Geometry check sheet. Reference: the model listing, model coordinates, mm. Face numbers are marked on the shaded views. Round coordinates to 2 decimals unless told otherwise and drop trailing zeros. Loops run counter-clockwise (first coordinate to the right, second up) from the corner with the lowest first, then second, coordinate; pieces in that order, holes last. Notation, with made-up numbers: (-20, -17.5) -> (12, -17.5) arc R23 cw to (12, 14.5) -> close; hole circle Ø10 at (75, -18). An arc over 180 degrees is marked (long way). Use a Markdown table: item, result. Add a question column.
Q1. Gauge pin test, flat ends, axial feed: P1, Ø6, axis at x = 12, z = 14.5, coming from the -Y side; P2, Ø13, axis at x = 5, y = 28, coming from the +Z side; P3, Ø8, axis at x = 25, y = 32.5, coming from the +Z side. Record the tip position at first contact, or that the pin passes through.
Q2. Sectioned sample at B-B, the plane z = 2. Enter the section's corners in (x, y).
Q3. Release check for a two-part mould opening along Y. For the marked faces 1, 2, 3 and 4 record: released by +Y, released by -Y, zero draft, split by the parting line, or undercut.
Q4. Sectioned sample at A-A, the plane x = 15. Enter the section's corners in (y, z), then the cut area to 3 significant figures.
Q5. Material ranges on L1, parallel to Z at x = 15, y = 33.5; L2, parallel to Y at x = 5, z = 1.5; L3, parallel to Y at x = 14, z = 15, recorded low to high.
Q6. Sectioned sample at D-D, the plane z = 19. Enter the section's corners in (x, y), then the cut area to 3 significant figures.
Q7. Sectioned sample at C-C, the plane y = 32. Enter the section's corners in (x, z), then the cut area to 3 significant figures.
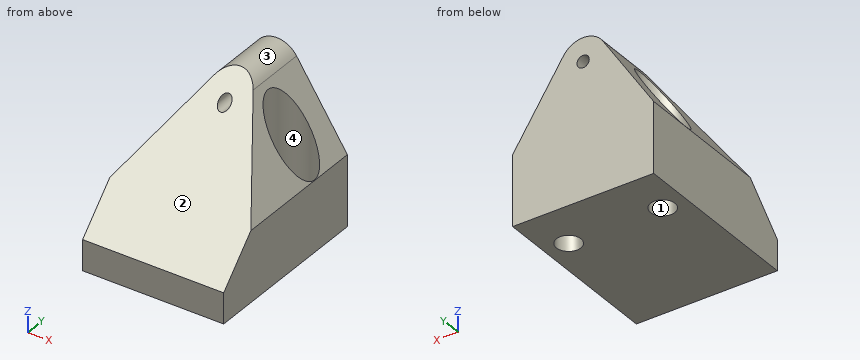
```python
from build123d import *

# Parameters (mm, degrees)
BOSS_EXTRUDE1_DEPTH = 30
CUT_EXTRUDE1_REACH  = 37
SKETCH3_R           = 2.6
CUT_EXTRUDE2_REACH  = 43.5
CUT_EXTRUDE2_START  = -6.5
SKETCH4_R           = 4.95
CUT_EXTRUDE3_REACH  = 40
SKETCH5_R           = 1.3
CUT_EXTRUDE4_REACH  = 40


with BuildPart() as part:
    # Sketch2 → Boss-Extrude1 (new body)
    with BuildSketch(Plane(origin=(0, 0, 0), x_dir=(0, 0, -1), z_dir=(1, 0, 0))):
        Polygon((0, 0), (-6.5, 0), (-35, 28), (-35, 38), (0, 38), align=None)
    extrude(amount=BOSS_EXTRUDE1_DEPTH)

    # Sketch3 → Cut-Extrude1 (cut, up to next)
    with BuildSketch(Plane(origin=(0, 0, 0), x_dir=(-1, 0, 0), z_dir=(0, 0, -1)), mode=Mode.PRIVATE) as cut_extrude1_sk1:
        with Locations((-25, 28)):
            Circle(SKETCH3_R)
    cut_extrude1_tool1 = extrude(cut_extrude1_sk1.sketch, amount=-CUT_EXTRUDE1_REACH, mode=Mode.PRIVATE) & part.part
    add(cut_extrude1_tool1.solids().sort_by_distance((25, 28, 0))[0], mode=Mode.SUBTRACT)
    # Sketch3 → Cut-Extrude1 (cut, up to next)
    with BuildSketch(Plane(origin=(0, 0, 0), x_dir=(-1, 0, 0), z_dir=(0, 0, -1)), mode=Mode.PRIVATE) as cut_extrude1_sk2:
        with Locations((-5, 28)):
            Circle(SKETCH3_R)
    cut_extrude1_tool2 = extrude(cut_extrude1_sk2.sketch, amount=-CUT_EXTRUDE1_REACH, mode=Mode.PRIVATE) & part.part
    add(cut_extrude1_tool2.solids().sort_by_distance((5, 28, 0))[0], mode=Mode.SUBTRACT)

    # Sketch4 → Cut-Extrude2 (cut, up to next)
    with BuildSketch(Plane(origin=(0, 0, 0), x_dir=(-1, 0, 0), z_dir=(0, 0, -1)).offset(CUT_EXTRUDE2_START), mode=Mode.PRIVATE) as cut_extrude2_sk1:
        with Locations((-25, 28)):
            Circle(SKETCH4_R)
    cut_extrude2_tool1 = extrude(cut_extrude2_sk1.sketch, amount=-CUT_EXTRUDE2_REACH, mode=Mode.PRIVATE) & part.part
    add(cut_extrude2_tool1.solids().sort_by_distance((25, 28, 6.5))[0], mode=Mode.SUBTRACT)
    # Sketch4 → Cut-Extrude2 (cut, up to next)
    with BuildSketch(Plane(origin=(0, 0, 0), x_dir=(-1, 0, 0), z_dir=(0, 0, -1)).offset(CUT_EXTRUDE2_START), mode=Mode.PRIVATE) as cut_extrude2_sk2:
        with Locations((-5, 28)):
            Circle(SKETCH4_R)
    cut_extrude2_tool2 = extrude(cut_extrude2_sk2.sketch, amount=-CUT_EXTRUDE2_REACH, mode=Mode.PRIVATE) & part.part
    add(cut_extrude2_tool2.solids().sort_by_distance((5, 28, 6.5))[0], mode=Mode.SUBTRACT)

    # Sketch5 → Cut-Extrude3 (cut, up to next)
    with BuildSketch(Plane(origin=(0, 38, 0), x_dir=(1, 0, 0), z_dir=(0, 1, 0)), mode=Mode.PRIVATE) as cut_extrude3_sk1:
        with Locations((15, -28.87)):
            Circle(SKETCH5_R)
    cut_extrude3_tool1 = extrude(cut_extrude3_sk1.sketch, amount=-CUT_EXTRUDE3_REACH, mode=Mode.PRIVATE) & part.part
    add(cut_extrude3_tool1.solids().sort_by_distance((15, 38, 28.87))[0], mode=Mode.SUBTRACT)

    # Sketch6 → Cut-Extrude4 (cut, up to next)
    with BuildSketch(Plane(origin=(0, 38, 0), x_dir=(1, 0, 0), z_dir=(0, 1, 0)), mode=Mode.PRIVATE) as cut_extrude4_sk1:
        with BuildLine():
            Line((0, -35), (30, -35))
            Line((30, -35), (30, -15))
            Line((30, -15), (19.189785955, -31.598679836))
            ThreePointArc((19.189785955, -31.598679836), (15, -33.87), (10.810214045, -31.598679836))
            Line((10.810214045, -31.598679836), (0, -15))
            Line((0, -15), (0, -35))
        make_face()
    cut_extrude4_tool1 = extrude(cut_extrude4_sk1.sketch, amount=-CUT_EXTRUDE4_REACH, mode=Mode.PRIVATE) & part.part
    add(cut_extrude4_tool1.solids().sort_by_distance((15, 38, 34.639445))[0], mode=Mode.SUBTRACT)


solid = part.part
```
Values:
| question | item | result |
|---|---|---|
| 1 | P1 | y = 4.91 |
| 1 | P2 | z = 32.44 |
| 1 | P3 | z = 28.82 |
| 2 | outline | (0, 0) -> (30, 0) -> (30, 38) -> (0, 38) -> close; hole circle Ø5.2 at (5, 28); hole circle Ø5.2 at (25, 28) |
| 3 | face 1 | undercut |
| 3 | face 2 | released by -Y |
| 3 | face 3 | zero draft |
| 3 | face 4 | undercut |
| 4 | outline | (0, 0) -> (38, 0) -> (38, 27.57) -> (20.7, 27.57) -> (0, 6.5) -> close; (23.25, 30.17) -> (38, 30.17) -> (38, 33.87) -> (26.89, 33.87) -> close |
| 4 | area | 877 mm^2 |
| 5 | L1 | 0 to 27.57, 30.17 to 33.87 |
| 5 | L2 | 0 to 25.4, 30.6 to 38 |
| 5 | L3 | 8.35 to 38 |
| 6 | outline | (2.61, 12.28) -> (27.39, 12.28) -> (27.39, 23.67) arc R4.95 cw (long way) to (27.39, 32.33) -> (27.39, 38) -> (2.61, 38) -> (2.61, 32.33) arc R4.95 cw (long way) to (2.61, 23.67) -> close |
| 6 | area | 515 mm^2 |
| 7 | outline | (0, 0) -> (30, 0) -> (30, 15) -> (27.92, 18.2) -> (27.92, 6.5) -> (22.08, 6.5) -> (22.08, 27.15) -> (19.19, 31.6) arc R5 ccw to (10.81, 31.6) -> (7.92, 27.15) -> (7.92, 6.5) -> (2.08, 6.5) -> (2.08, 18.2) -> (0, 15) -> close; hole circle Ø2.6 at (15, 28.87) |
| 7 | area | 588 mm^2 |
